Part print with two shaded views. Sizes in mm from the minimum x, y, z corner. Coordinates: 2 decimals unless noted, no trailing zeros. Loops run counter-clockwise (first coordinate to the right, second up) from the corner with the lowest first, then second, coordinate; pieces in that order, holes last.
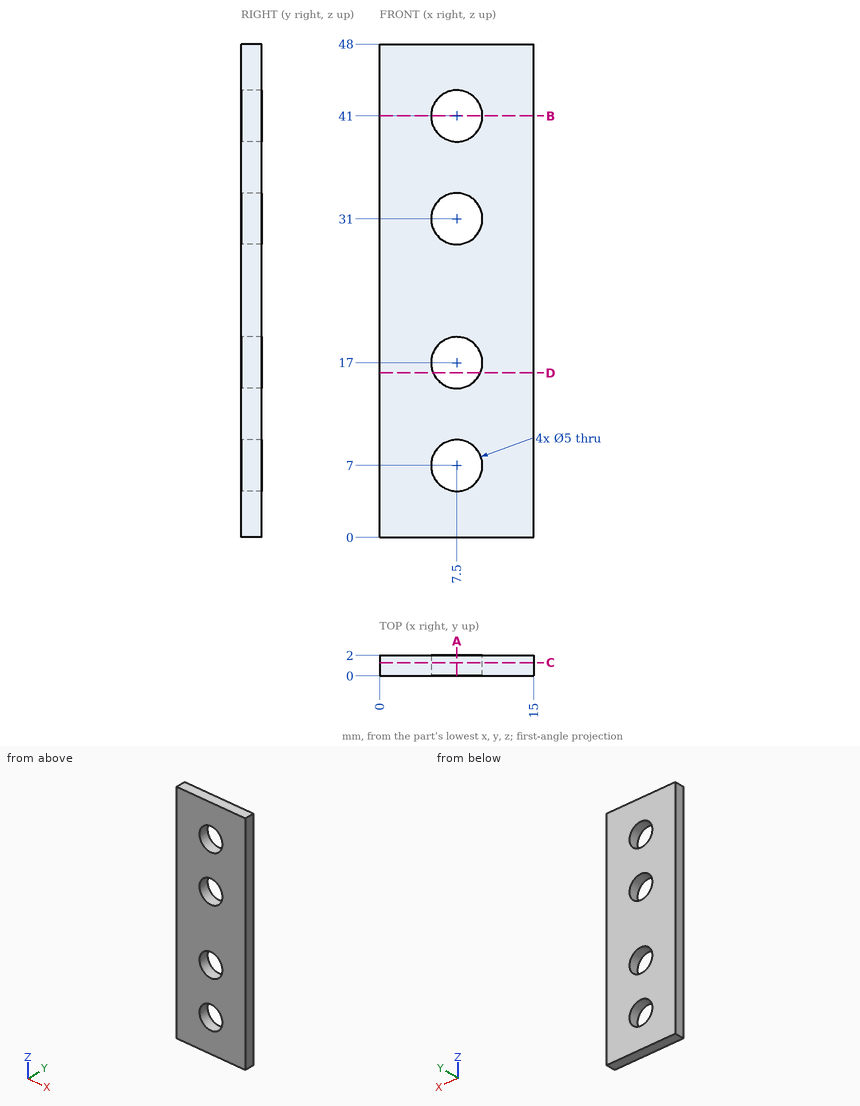
Q1. Slice it at A-A (x = 7.5). List the corners of the cut face in (y, z), and give its area (3 significant figures).
Answers:
outline: (0, 0) - (2, 0) - (2, 4.5) - (0, 4.5) - close; (0, 9.5) - (2, 9.5) - (2, 14.5) - (0, 14.5) - close; (0, 19.5) - (2, 19.5) - (2, 28.5) - (0, 28.5) - close; (0, 33.5) - (2, 33.5) - (2, 38.5) - (0, 38.5) - close; (0, 43.5) - (2, 43.5) - (2, 48) - (0, 48) - close
area: 56.0 mm2
Q2. Slice it at B-B (z = 41). List the corners of the cut face in (x, y), and give its area (3 significant figures).
Answers:
outline: (0, 0) - (5, 0) - (5, 2) - (0, 2) - close; (10, 0) - (15, 0) - (15, 2) - (10, 2) - close
area: 20.0 mm2
Q3. Slice it at D-D (z = 16). List the corners of the cut face in (x, y), and give its area (3 significant figures).
Answers:
outline: (0, 0) - (5.21, 0) - (5.21, 2) - (0, 2) - close; (9.79, 0) - (15, 0) - (15, 2) - (9.79, 2) - close
area: 20.8 mm2
Q4. Slice it at C-C (y = 1.3). List the corners of the cut face in (x, z).
Answers:
outline: (0, 0) - (15, 0) - (15, 48) - (0, 48) - close; hole circle Ø5 at (7.5, 7); hole circle Ø5 at (7.5, 17); hole circle Ø5 at (7.5, 31); hole circle Ø5 at (7.5, 41)
Q5. Drill centre lines: line 1 (Z direction, x = 7.5, y = 1.25); line 2 (Z direction, x = 8.5, y = 1.5); line 3 (X direction, y = 0.9, z = 39). Where is each one in solid material? Low to high.
Answers:
line 1: z = 0 to 4.5, 9.5 to 14.5, 19.5 to 28.5, 33.5 to 38.5, 43.5 to 48
line 2: z = 0 to 4.71, 9.29 to 14.71, 19.29 to 28.71, 33.29 to 38.71, 43.29 to 48
line 3: x = 0 to 6, 9 to 15
Q6. Flat gauge pins, fed straight in: P1, Ø1.5, axis at x = 3.5, z = 34, coming from the -Y side; P2, Ø4.5, axis at x = 7.5, z = 31, coming from the +Y side. Where does each tip first touch, or does it go through?
Answers:
P1: stops at y = 0
P2: passes through
